Verification items for the finished model (mm, model axes). A direction names the side the tool comes from. Round coordinates to 2 decimals unless told otherwise and drop trailing zeros. Loops run counter-clockwise (first coordinate to the right, second up) from the corner with the lowest first, then second, coordinate; pieces in that order, holes last.
from build123d import *

# Parameters (mm, degrees)
F0_W     = 80
F0_H     = 82
F1_DEPTH = 4
F2_W     = 80
F2_H     = 82
F3_DEPTH = 36


with BuildPart() as f1:
    # F0 (on Top) → F1 (new body)
    with BuildSketch(Plane.XY):
        Rectangle(F0_W, F0_H)
    extrude(amount=F1_DEPTH)

    # F2 (on face) → F3 (join)
    with BuildSketch(Plane.XY.offset(4)):
        Rectangle(F2_W, F2_H)
        Polygon((-37, 29.3), (-19.3, 29.3), (-19.3, 38), (19.3, 38), (19.3, 29.3), (37, 29.3), (37, -29.3), (19.3, -29.3), (19.3, -38), (-19.3, -38), (-19.3, -29.3), (-37, -29.3), align=None, mode=Mode.SUBTRACT)
    extrude(amount=F3_DEPTH)


solid = f1.part
1. Tool access check on faces 5 (the face through (-28, 29.3, 22)), 6 (the face through (40, -1, 20)). Record the directions out of +Z, -Z, +X, -X, +Y, -Y that give a thin tool (end or side, any length) a straight path to the whole face; none if there is none.
2. Release check for a two-part mould opening along X. For faces 1 (the face through (-1, 41, 20)), 2 (the face through (-40, -1, 20)), 3 (the face through (-37, 0, 22)), 4 (the face through (-1, 1, 4)) record: released by +X, released by -X, zero draft, split by the parting line, or undercut.
3. Gauge pin test, flat end, axial feed: P1, Ø6, axis at x = -4, y = -22, coming from the +Z side. Record the tip position at first contact, or that the pin passes through.
4. Section check B-B (x = -4). Enter the section's corners in (y, z).
5. Section check C-C (y = -3). Enter the section's corners in (x, z).
6. Section check A-A (z = 9). Enter the section's corners in (x, y).
7. Scan lines: L1, parallel to Y at x = 27.5, z = 9; L2, parallel to Y at x = -11, z = 10; L3, parallel to X at y = -14, z = 35.5. Record each from-to range of solid material in increasing order.
Taken from the geometry:
1. face 5: +Z
1. face 6: +Z, -Z, +X, +Y, -Y
2. face 1: zero draft
2. face 2: released by -X
2. face 3: undercut
2. face 4: undercut
3. P1: stops at z = 4
4. outline: (-41, 0) - (41, 0) - (41, 40) - (38, 40) - (38, 4) - (-38, 4) - (-38, 40) - (-41, 40) - close
5. outline: (-40, 0) - (40, 0) - (40, 40) - (37, 40) - (37, 4) - (-37, 4) - (-37, 40) - (-40, 40) - close
6. outline: (-40, -41) - (40, -41) - (40, 41) - (-40, 41) - close; hole (-37, -29.3) - (-19.3, -29.3) - (-19.3, -38) - (19.3, -38) - (19.3, -29.3) - (37, -29.3) - (37, 29.3) - (19.3, 29.3) - (19.3, 38) - (-19.3, 38) - (-19.3, 29.3) - (-37, 29.3) - close
7. L1: y = -41 to -29.3, 29.3 to 41
7. L2: y = -41 to -38, 38 to 41
7. L3: x = -40 to -37, 37 to 40
